Geometry check sheet. Reference: drawing and pictorial views, mm from the part's lowest x, y, z. Give positions to 0.01 mm unless a question says otherwise; leave off trailing zeros. Order: outer loops, then holes, each group sorted by start corner. A loop starts at its lowest first (then second) coordinate and runs counter-clockwise, first axis right, second up.
Item 1: Sectioned sample at A-A on z = 2.25. Record the boundary of the cut face in (x, y), and give its area (3 significant figures).
Item 2: Gauge pin test, flat ends, axial feed: P1, Ø1.2, axis at x = 11, y = 1.5, coming from the -Z side; P2, Ø1.2, axis at y = 2.5, z = 2.5, coming from the +X side. Record the tip position at first contact, or that the pin passes through.
Item 3: Material ranges on line 1 along X through (y, z) = (3.8, 3); line 2 along Z through (x, y) = (96, 2.75); line 3 along X through (y, z) = (0.7, 10.5), recorded low to high.
Item 4: Sectioned sample at C-C on z = 10.5. Record the boundary of the cut face in (x, y).
Item 5: Sectioned sample at B-B on x = 115.5. Record the boundary of the cut face in (y, z), and give its area (3 significant figures).
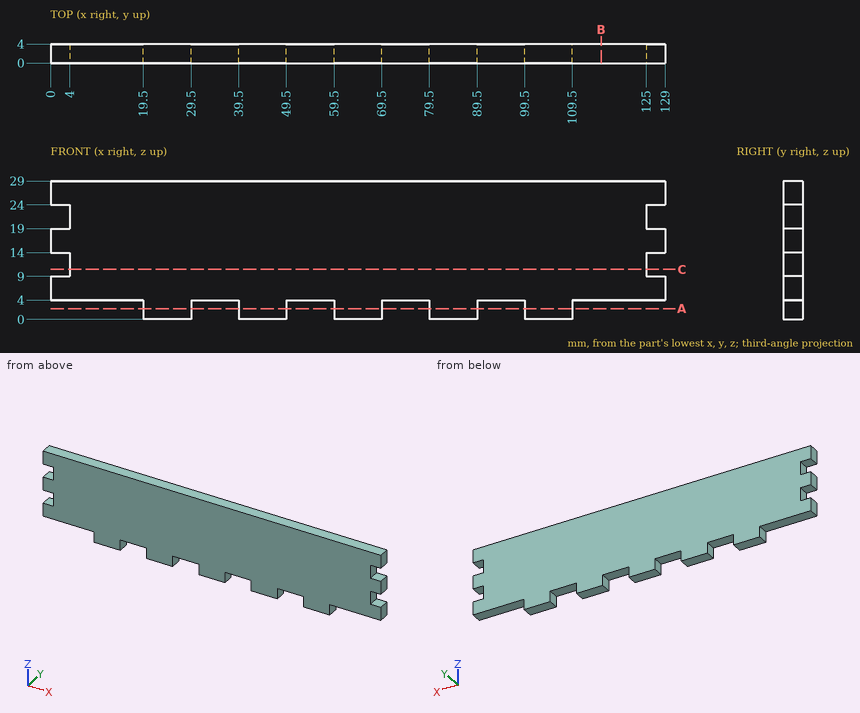
Report:
1. outline: (19.5, 0) - (29.5, 0) - (29.5, 4) - (19.5, 4) - close; (39.5, 0) - (49.5, 0) - (49.5, 4) - (39.5, 4) - close; (59.5, 0) - (69.5, 0) - (69.5, 4) - (59.5, 4) - close; (79.5, 0) - (89.5, 0) - (89.5, 4) - (79.5, 4) - close; (99.5, 0) - (109.5, 0) - (109.5, 4) - (99.5, 4) - close
1. area: 200 mm2
2. P1: stops at z = 4
2. P2: stops at x = 109.5
3. line 1: x = 19.5 to 29.5, 39.5 to 49.5, 59.5 to 69.5, 79.5 to 89.5, 99.5 to 109.5
3. line 2: z = 4 to 29
3. line 3: x = 4 to 125
4. outline: (4, 0) - (125, 0) - (125, 4) - (4, 4) - close
5. outline: (0, 4) - (4, 4) - (4, 29) - (0, 29) - close
5. area: 100 mm2
